The model under review builds one solid part; all positions refer to its coordinate system, in mm. A direction names the side the tool comes from. Coordinates: 2 decimals unless noted, no trailing zeros. Write each loop counter-clockwise with the first axis right and the second up, starting at its lowest first coordinate (ties: lowest second). Pieces come first, ordered by that corner, then holes.
```python
from build123d import *

# Parameters (mm, degrees)
SKETCH1_R               = 7.5
BOSS_EXTRUDE1_DEPTH     = 50.5
SKETCH2_W               = 2
SKETCH2_H               = 3.5
CUT_EXTRUDE1_DEPTH      = 1.5
SKETCH3_W               = 3.5
SKETCH3_H               = 2
CUT_EXTRUDE2_DEPTH      = 1.5
SKETCH4_W               = 3.5
SKETCH4_H               = 2
CUT_EXTRUDE3_DEPTH      = 1.5
SKETCH5_W               = 3.5
SKETCH5_H               = 3.854101966
CUT_EXTRUDE4_DEPTH      = 6.25
MIRROR3_COPY_1_SKETCH_W = 2
MIRROR3_COPY_1_SKETCH_H = 3.5
MIRROR3_COPY_1_DEPTH    = 1.5
MIRROR3_COPY_2_SKETCH_W = 3.5
MIRROR3_COPY_2_SKETCH_H = 2
MIRROR3_COPY_2_DEPTH    = 1.5
MIRROR3_COPY_3_SKETCH_W = 3.5
MIRROR3_COPY_3_SKETCH_H = 2
MIRROR3_COPY_3_DEPTH    = 1.5
MIRROR3_COPY_4_SKETCH_W = 3.5
MIRROR3_COPY_4_SKETCH_H = 3.854101966
MIRROR3_COPY_4_DEPTH    = 6.25


with BuildPart() as part:
    # Sketch1 → Boss-Extrude1 (new body)
    with BuildSketch(Plane.XY):
        with BuildLine():
            Line((0, 9), (39, 9))
            ThreePointArc((39, 9), (46.794228634, 4.5), (46.794228634, -4.5))
            Line((46.794228634, -4.5), (37.044228634, -21.387495374))
            ThreePointArc((37.044228634, -21.387495374), (33.75, -24.681724008), (29.25, -25.887495374))
            Line((29.25, -25.887495374), (9.75, -25.887495374))
            ThreePointArc((9.75, -25.887495374), (5.25, -24.681724008), (1.955771366, -21.387495374))
            Line((1.955771366, -21.387495374), (-7.794228634, -4.5))
            ThreePointArc((-7.794228634, -4.5), (-7.794228634, 4.5), (0, 9))
        make_face()
        with Locations(Location((0, 0, 0), (0, 0, 180))):
            Circle(SKETCH1_R, mode=Mode.SUBTRACT)
        with Locations(Location((9.75, -16.887495374, 0), (0, 0, 180))):
            Circle(SKETCH1_R, mode=Mode.SUBTRACT)
        with Locations(Location((19.5, 0, 0), (0, 0, 180))):
            Circle(SKETCH1_R, mode=Mode.SUBTRACT)
        with Locations(Location((39, 0, 0), (0, 0, 180))):
            Circle(SKETCH1_R, mode=Mode.SUBTRACT)
        with Locations(Location((29.25, -16.887495374, 0), (0, 0, 180))):
            Circle(SKETCH1_R, mode=Mode.SUBTRACT)
    extrude(amount=BOSS_EXTRUDE1_DEPTH)

    # Sketch2 → Cut-Extrude1 (cut)
    with BuildSketch(Plane(origin=(37.044228634, -21.387495374, 0), x_dir=(0, 0, -1), z_dir=(0.8660254037844384, -0.5000000000000007, 0))):
        with Locations((-5.25, 9.75)):
            Rectangle(SKETCH2_W, SKETCH2_H)
    cut_extrude1 = extrude(amount=-CUT_EXTRUDE1_DEPTH, mode=Mode.SUBTRACT)

    # Sketch3 → Cut-Extrude2 (cut)
    with BuildSketch(Plane(origin=(0, 9, 0), x_dir=(1, 0, 0), z_dir=(0, 1, 0))):
        with Locations((29.25, -5.25)):
            Rectangle(SKETCH3_W, SKETCH3_H)
    cut_extrude2 = extrude(amount=-CUT_EXTRUDE2_DEPTH, mode=Mode.SUBTRACT)

    # Sketch4 → Cut-Extrude3 (cut)
    with BuildSketch(Plane.XZ.offset(25.887495374)):
        with Locations((19.5, 5.25)):
            Rectangle(SKETCH4_W, SKETCH4_H)
    cut_extrude3 = extrude(amount=-CUT_EXTRUDE3_DEPTH, mode=Mode.SUBTRACT)

    # Sketch5 → Cut-Extrude4 (cut)
    with BuildSketch(Plane(origin=(0, 0, 0), x_dir=(-1, 0, 0), z_dir=(0, 0, -1))):
        with Locations((-29.25, 5.822949017)):
            Rectangle(SKETCH5_W, SKETCH5_H)
        with Locations((-19.5, -22.710444391)):
            Rectangle(SKETCH5_W, SKETCH5_H)
        Polygon((-38.373946668, -8.876152247), (-36.623946668, -11.90724116), (-39.961696879, -13.834292144), (-41.711696879, -10.80320323), align=None)
    cut_extrude4 = extrude(amount=-CUT_EXTRUDE4_DEPTH, mode=Mode.SUBTRACT)

    # Mirror2: Cut-Extrude1, Cut-Extrude2, Cut-Extrude3, Cut-Extrude4 across plane
    add(cut_extrude1.mirror(Plane(origin=(19.5, 0, 0), x_dir=(0, 0, 1), z_dir=(1, 0, 0))), mode=Mode.SUBTRACT)
    add(cut_extrude2.mirror(Plane(origin=(19.5, 0, 0), x_dir=(0, 0, 1), z_dir=(1, 0, 0))), mode=Mode.SUBTRACT)
    add(cut_extrude3.mirror(Plane(origin=(19.5, 0, 0), x_dir=(0, 0, 1), z_dir=(1, 0, 0))), mode=Mode.SUBTRACT)
    add(cut_extrude4.mirror(Plane(origin=(19.5, 0, 0), x_dir=(0, 0, 1), z_dir=(1, 0, 0))), mode=Mode.SUBTRACT)

    # Mirror3: Cut-Extrude1, Cut-Extrude2, Cut-Extrude3, Cut-Extrude4 across plane
    add(cut_extrude1.mirror(Plane(origin=(0, 0, 25.25), x_dir=(1, 0, 0), z_dir=(0, 0, -1))), mode=Mode.SUBTRACT)
    add(cut_extrude2.mirror(Plane(origin=(0, 0, 25.25), x_dir=(1, 0, 0), z_dir=(0, 0, -1))), mode=Mode.SUBTRACT)
    add(cut_extrude3.mirror(Plane(origin=(0, 0, 25.25), x_dir=(1, 0, 0), z_dir=(0, 0, -1))), mode=Mode.SUBTRACT)
    add(cut_extrude4.mirror(Plane(origin=(0, 0, 25.25), x_dir=(1, 0, 0), z_dir=(0, 0, -1))), mode=Mode.SUBTRACT)

    # Mirror3 copy 1 sketch → Mirror3 copy 1 (cut)
    with BuildSketch(Plane(origin=(1.955771366, -21.387495374, 50.5), x_dir=(0, 0, 1), z_dir=(-0.8660254037844385, -0.5000000000000004, 0))):
        with Locations((-5.25, 9.75)):
            Rectangle(MIRROR3_COPY_1_SKETCH_W, MIRROR3_COPY_1_SKETCH_H)
    extrude(amount=-MIRROR3_COPY_1_DEPTH, mode=Mode.SUBTRACT)

    # Mirror3 copy 2 sketch → Mirror3 copy 2 (cut)
    with BuildSketch(Plane(origin=(39, 9, 50.5), x_dir=(-1, 0, 0), z_dir=(0, 1, 0))):
        with Locations((29.25, -5.25)):
            Rectangle(MIRROR3_COPY_2_SKETCH_W, MIRROR3_COPY_2_SKETCH_H)
    extrude(amount=-MIRROR3_COPY_2_DEPTH, mode=Mode.SUBTRACT)

    # Mirror3 copy 3 sketch → Mirror3 copy 3 (cut)
    with BuildSketch(Plane(origin=(39, -25.887495374, 50.5), x_dir=(-1, 0, 0), z_dir=(0, -1, 0))):
        with Locations((19.5, 5.25)):
            Rectangle(MIRROR3_COPY_3_SKETCH_W, MIRROR3_COPY_3_SKETCH_H)
    extrude(amount=-MIRROR3_COPY_3_DEPTH, mode=Mode.SUBTRACT)

    # Mirror3 copy 4 sketch → Mirror3 copy 4 (cut)
    with BuildSketch(Plane(origin=(39, 0, 50.5), x_dir=(1, 0, 0), z_dir=(0, 0, 1))):
        with Locations((-29.25, 5.822949017)):
            Rectangle(MIRROR3_COPY_4_SKETCH_W, MIRROR3_COPY_4_SKETCH_H)
        with Locations((-19.5, -22.710444391)):
            Rectangle(MIRROR3_COPY_4_SKETCH_W, MIRROR3_COPY_4_SKETCH_H)
        Polygon((-38.373946668, -8.876152247), (-36.623946668, -11.90724116), (-39.961696879, -13.834292144), (-41.711696879, -10.80320323), align=None)
    extrude(amount=-MIRROR3_COPY_4_DEPTH, mode=Mode.SUBTRACT)


solid = part.part
```
Item 1: Take a section at C-C, the plane y = -23. Write out the cut boundary in (x, z), plus the area to 3 significant figures.
Solved:
outline: (3.14, 0) - (5.4, 0) - (5.4, 50.5) - (3.14, 50.5) - close; (14.1, 0) - (17.75, 0) - (17.75, 6.25) - (21.25, 6.25) - (21.25, 0) - (24.9, 0) - (24.9, 50.5) - (21.25, 50.5) - (21.25, 44.25) - (17.75, 44.25) - (17.75, 50.5) - (14.1, 50.5) - close; (33.6, 0) - (35.86, 0) - (35.86, 50.5) - (33.6, 50.5) - close
area: 730 mm2
Item 2: To check wall thickness, follow line 1 along Y through (x, z) = (29, 15); line 2 along Y through (x, z) = (19.5, 30.5); line 3 along Y through (x, z) = (25.5, 25). State the ranges of each line that lie inside material, in increasing order.
Solved:
line 1: y = -25.89 to -24.38, -9.39 to 9
line 2: y = -25.89 to -7.5, 7.5 to 9
line 3: y = -25.89 to -23.38, -10.39 to -4.5, 4.5 to 9
Item 3: For pin 1 (9 mm diameter, centred on x = 39, y = 0, fed in from -Z); pin 2 (1.5 mm diameter, centred on y = 7, z = 47.5, fed in from +X); pin 3 (2.5 mm diameter, centred on y = 6, z = 47.5, fed in from -X); pin 4 (1.5 mm diameter, centred on y = 5.5, z = 4, fed in from +X), all flat-tipped, find the tip position at first contact; note any pin that passes through.
Solved:
pin 1: passes through
pin 2: stops at x = 45.48
pin 3: stops at x = -7.64
pin 4: stops at x = 46.64
Item 4: Machinability: for faces 3 (the face through (10, 3.896, 3)), 4 (the face through (10, 7.75, 48)), 5 (the face through (19, 9, 25)), 6 (the face through (10, 6, 44.25)), 7 (the face through (36.743, -17.217, 24.896)), which of the approach directions +Z, -Z, +X, -X, +Y, -Y give a long, thin tool a straight path to every point of the face, cutting with its end or side? Answer none if there is none.
Solved:
face 3: -Z
face 4: +Z
face 5: +Z, -Z, +X, -X, +Y
face 6: +Y
face 7: +Z, -Z
Item 5: Take a section at D-D, the plane z = 20. Write out the cut boundary in (x, y).
Solved:
outline: (-7.79, -4.5) - (1.96, -21.39) arc R9 ccw to (9.75, -25.89) - (29.25, -25.89) arc R9 ccw to (37.04, -21.39) - (46.79, -4.5) arc R9 ccw to (39, 9) - (0, 9) arc R9 ccw to start; hole circle Ø15 at (0, 0); hole circle Ø15 at (9.75, -16.89); hole circle Ø15 at (19.5, 0); hole circle Ø15 at (29.25, -16.89); hole circle Ø15 at (39, 0)
Item 6: Take a section at A-A, the plane y = 0. Write out the cut boundary in (x, z).
Solved:
outline: (-9, 0) - (-7.5, 0) - (-7.5, 50.5) - (-9, 50.5) - close; (7.5, 0) - (12, 0) - (12, 50.5) - (7.5, 50.5) - close; (27, 0) - (31.5, 0) - (31.5, 50.5) - (27, 50.5) - close; (46.5, 0) - (48, 0) - (48, 50.5) - (46.5, 50.5) - close
Item 7: Mouldability with a two-part tool opening along Z and no side actions: class faces 1 (the face through (10, 6, 6.25)), 2 (the face through (10, 3.896, 47)) as pulls with the +Z half, pulls with the -Z half, needs draft (parallel to the pull), parting line crosses it, or undercut.
Solved:
face 1: undercut
face 2: needs draft
Item 8: Take a section at B-B, the plane x = 19.5. Write out the cut boundary in (y, z), plus the area to 3 significant figures.
Solved:
outline: (-25.89, 0) - (-24.64, 0) - (-24.64, 4.25) - (-25.89, 4.25) - close; (-25.89, 6.25) - (-20.78, 6.25) - (-20.78, 0) - (-7.5, 0) - (-7.5, 50.5) - (-20.78, 50.5) - (-20.78, 44.25) - (-25.89, 44.25) - close; (-25.89, 46.25) - (-24.64, 46.25) - (-24.64, 50.5) - (-25.89, 50.5) - close; (7.5, 0) - (9, 0) - (9, 50.5) - (7.5, 50.5) - close
area: 951 mm2
